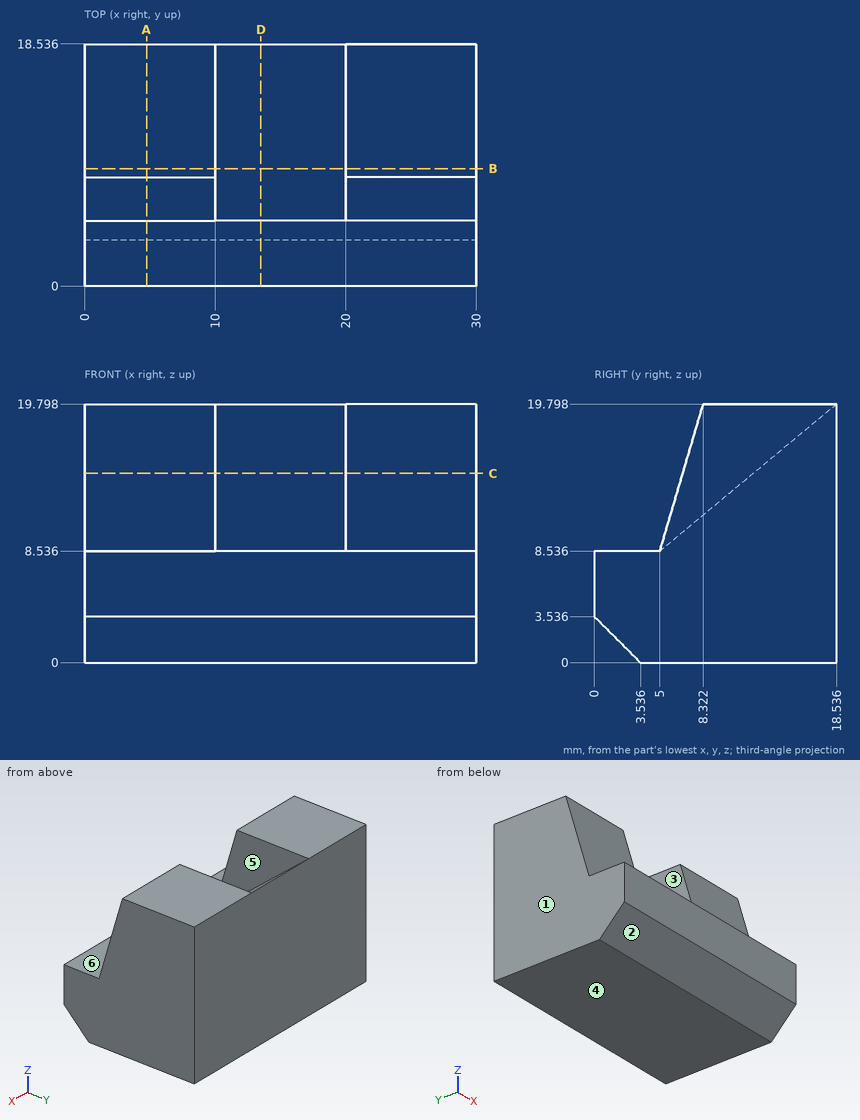
Job drawing, mm, ordinate dimensions from the low corner. One solid piece. A direction names the side the tool comes from. Give positions to 0.01 mm unless a question says otherwise; leave off trailing zeros. Write each loop counter-clockwise with the first axis right and the second up, starting at its lowest first coordinate (ties: lowest second). Pieces come first, ordered by that corner, then holes. Notation, with made-up numbers: M 46,20 L 69,20 A8 ccw 69,32 Z; hole C 33,17 d9. An arc over 180 degrees is marked long. Put each result on its own line as item: value. Start each with the question number.
(1) Probe L1, parallel to X at y = 10.5, z = 19.25; L2, parallel to Z at x = 2.25, y = 4 (1 decimal); L3, parallel to Y at x = 21.25, z = 13.25 (1 decimal). List the from-to ranges inside material, lowest first.
(2) Band-saw the part on C-C, the plane z = 14.5. Write the cut outline in (x, y) (1 decimal), and give its area (3 significant figures).
(3) Flat gauge pins, fed straight in: pin 1 Ø2.5 at (x, y) = (19.5, 3.5) entering from +Z; pin 2 Ø2 at (x, z) = (16, 5) entering from -Y. Where does each tip first touch, or does it go through?
(4) Which spindle directions (+Z, -Z, +X, -X, +Y, -Y) get a long thin tool onto all of the face, cutting with end or side? Do the marked faces 4, 5 and 6. Say none if no direction does.
(5) Mould opens along X. For the marked faces 1, 2 and 3 say: +X half, -X half, draft (parallel to the pull), parting line (faces both ways), or undercut.
(6) Band-saw the part on A-A, the plane x = 4.75. Write the cut outline in (y, z) (1 decimal).
(7) Band-saw the part on D-D, the plane x = 13.5. Write the cut outline in (y, z) (1 decimal).
(8) Band-saw the part on B-B, the plane y = 9. Write the cut outline in (x, z).
Response values:
1. L1: x = 0 to 10, 20 to 30
1. L2: z = 0 to 8.5
1. L3: y = 6.4 to 18.5
2. outline: M 0,6.8 L 10,6.8 L 10,12.2 L 20,12.2 L 20,6.8 L 30,6.8 L 30,18.5 L 0,18.5 Z
2. area: 299 mm2
3. pin 1: stops at z = 8.54
3. pin 2: stops at y = 0
4. face 4: -Z, +X, -X, +Y, -Y
4. face 5: +Z, -Y
4. face 6: +Z, +X, -X, -Y
5. face 1: -X half
5. face 2: draft
5. face 3: undercut
6. outline: M 0,3.5 L 3.5,0 L 18.5,0 L 18.5,19.8 L 8.3,19.8 L 5,8.5 L 0,8.5 Z
7. outline: M 0,3.5 L 3.5,0 L 18.5,0 L 18.5,19.8 L 5,8.5 L 0,8.5 Z
8. outline: M 0,0 L 30,0 L 30,19.8 L 20,19.8 L 20,11.86 L 10,11.86 L 10,19.8 L 0,19.8 Z
